Could you check a few things on this model? Use its own coordinates, in mm. Face numbers are marked on the shaded views. A direction names the side the tool comes from. Give positions to 0.01 mm unless a question says otherwise; leave off trailing zeros. Write each loop counter-clockwise with the first axis right and the second up, starting at its lowest first coordinate (ties: lowest second). Pieces come first, ordered by that corner, then holes. Notation, with made-up numbers: (-19.5, 3) - (-15.5, 3) arc R12 cw to (-15.5, 18) - close; hole circle Ø6 at (85.25, 82.25). An arc over 180 degrees is marked (long way). Use one line per item in the form item = value.
```python
from build123d import *

# Parameters (mm, degrees)
SKETCH_1_R          = 6
SKETCH_1_R_2        = 1.5
SKETCH_1_W          = 40
SKETCH_1_H          = 1.5
EXTRUDE_1_DEPTH     = 1.5
SKETCH_1_3_W        = 40
SKETCH_1_3_H        = 1.5
EXTRUDE_2_DEPTH     = 40
SKETCH_2_R          = 1.5
CUT_EXTRUDE_1_DEPTH = 2.5


with BuildPart() as part:
    # Sketch 1 → Extrude 1 (new body)
    with BuildSketch(Plane.XY):
        with BuildLine():
            Line((20, 0), (20, -25))
            Line((20, -25), (-20, -25))
            Line((-20, -25), (-20, 0))
            ThreePointArc((-20, 0), (0, 20), (20, 0))
        make_face()
        with Locations((0, 7)):
            Circle(SKETCH_1_R, mode=Mode.SUBTRACT)
        with Locations((-15.5, 0)):
            Circle(SKETCH_1_R_2, mode=Mode.SUBTRACT)
        with Locations((-7.75, 13.423393759)):
            Circle(SKETCH_1_R_2, mode=Mode.SUBTRACT)
        with Locations((7.75, 13.423393759)):
            Circle(SKETCH_1_R_2, mode=Mode.SUBTRACT)
        with Locations((15.5, 0)):
            Circle(SKETCH_1_R_2, mode=Mode.SUBTRACT)
        with Locations((7.75, -13.423393759)):
            Circle(SKETCH_1_R_2, mode=Mode.SUBTRACT)
        with Locations((-7.75, -13.423393759)):
            Circle(SKETCH_1_R_2, mode=Mode.SUBTRACT)
        with Locations((0, -24.25)):
            Rectangle(SKETCH_1_W, SKETCH_1_H)
    extrude(amount=EXTRUDE_1_DEPTH)

    # Sketch 1_3 → Extrude 2 (add)
    with BuildSketch(Plane.XY):
        with Locations((0, -24.25)):
            Rectangle(SKETCH_1_3_W, SKETCH_1_3_H)
    extrude(amount=-EXTRUDE_2_DEPTH)

    # Sketch 2 → Cut-Extrude 1 (cut, through all)
    with BuildSketch(Plane(origin=(0, -23.5, 0), x_dir=(1, 0, 0), z_dir=(0, 1, 0))):
        with Locations((-14.75, 31.95)):
            Circle(SKETCH_2_R)
        with Locations((-14.75, 7.75)):
            Circle(SKETCH_2_R)
        with Locations((14.75, 7.75)):
            Circle(SKETCH_2_R)
        with Locations((14.75, 31.95)):
            Circle(SKETCH_2_R)
    extrude(amount=-CUT_EXTRUDE_1_DEPTH, mode=Mode.SUBTRACT)


solid = part.part
```
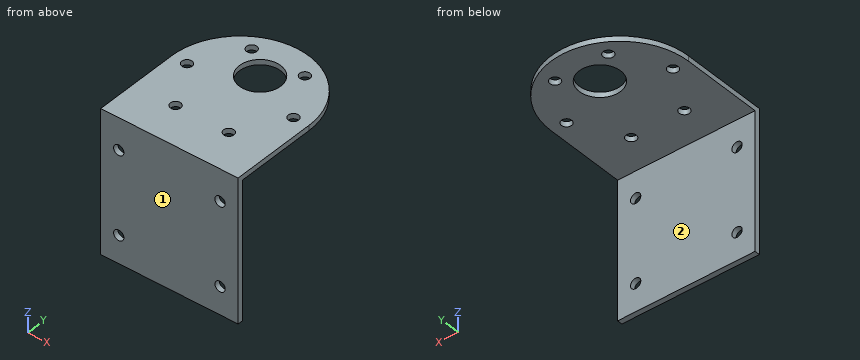
1. For pin 1 (5 mm diameter, centred on x = 10.5, y = -5, fed in from -Z); pin 2 (4 mm diameter, centred on x = 12, z = -33, fed in from +Y), each with a flat end and sliding along its axis, tell me the tip position at first contact or that it passes through.
Response values:
pin_1 = 0
pin_2 = -23.5
2. Imagine slicing it at B-B, the plane x = 0. List the corners of the cut face in (y, z) for me.
Response values:
outline = (-25, -40) - (-23.5, -40) - (-23.5, 0) - (1, 0) - (1, 1.5) - (-25, 1.5) - close; (13, 0) - (20, 0) - (20, 1.5) - (13, 1.5) - close
3. If I drill on line 1 (Z direction, x = -14.75, y = -24.2); line 2 (Z direction, x = 1.5, y = -7); line 3 (Y direction, x = 13, z = -12), over which ranges is the centre line in solid material (lowest first)? Write a range as from..to.
Response values:
line_1 = -40..-33.45, -30.45..-9.25, -6.25..1.5
line_2 = 0..1.5
line_3 = -25..-23.5
4. Which directions (+Z, -Z, +X, -X, +Y, -Y) give clear straight access to the entire face, cutting with the end or side of a thin tool? Please do the marked faces 1 and 2.
Response values:
face_1 = +Z, -Z, +X, -X, -Y
face_2 = -Z, +X, -X, +Y
5. Imagine slicing it at C-C, the plane y = 7. List the corners of the cut face in (x, z) for me (3 decimals).
Response values:
outline = (-18.735, 0) - (-6, 0) - (-6, 1.5) - (-18.735, 1.5) - close; (6, 0) - (18.735, 0) - (18.735, 1.5) - (6, 1.5) - close
6. Imagine slicing it at D-D, the plane x = 14.75. List the corners of the cut face in (y, z) for me, and give its area (3 significant figures).
Response values:
outline = (-25, -40) - (-23.5, -40) - (-23.5, -33.45) - (-25, -33.45) - close; (-25, -30.45) - (-23.5, -30.45) - (-23.5, -9.25) - (-25, -9.25) - close; (-25, -6.25) - (-23.5, -6.25) - (-23.5, 0) - (-1.3, 0) - (-1.3, 1.5) - (-25, 1.5) - close; (1.3, 0) - (13.51, 0) - (13.51, 1.5) - (1.3, 1.5) - close
area = 105 mm²
7. Imagine slicing it at A-A, the plane z = -31.95. List the corners of the cut face in (x, y) for me, and give its area (3 significant figures).
Response values:
outline = (-20, -25) - (-16.25, -25) - (-16.25, -23.5) - (-20, -23.5) - close; (-13.25, -25) - (13.25, -25) - (13.25, -23.5) - (-13.25, -23.5) - close; (16.25, -25) - (20, -25) - (20, -23.5) - (16.25, -23.5) - close
area = 51.0 mm²
